Source: three-view drawing plus pictorial views. Frame: mm from the lowest corner of the part. A direction names the side the tool comes from. Coordinates: 2 decimals unless noted, no trailing zeros. Order: outer loops, then holes, each group sorted by start corner. A loop starts at its lowest first (then second) coordinate and runs counter-clockwise, first axis right, second up. Notation, with made-up numbers: (69, -27.75) -> (84, -27.75) arc R15 ccw to (84, -15.75) -> close; hole circle Ø11 at (3, 19). An arc over 180 degrees is marked (long way). Use one line per item in the form item = value. Start each with the question number.
1) Pin query (flat end, axial travel): pin 1 (4 mm diameter, centred on y = 4.5, z = 7, fed in from -X); pin 2 (6.5 mm diameter, centred on x = 9.5, y = 7, fed in from +Z); pin 3 (2 mm diameter, centred on x = 5.5, z = 3, fed in from +Y); pin 4 (5 mm diameter, centred on y = 12.5, z = 4, fed in from +X). Return the tip coordinate at first contact, or that it passes through.
2) Ray query, line 1 along Y through (x, z) = (8, 9.5); line 2 along Z through (x, y) = (2, 12.25); line 3 along Z through (x, y) = (4.25, 7.25). Return the intervals inside material, ascending.
3) Access query for the marked faces 4 and 5. Directions: +Z, -Z, +X, -X, +Y, -Y. A direction counts if a zero-diameter tool reaches every point of the face in a straight line with its end or side. Return the directions, or none.
4) Section query C-C on z = 8. Output: boundary loops of the cut face in (x, y), then the cut area to 3 significant figures.
5) Draft query along X for the marked faces 1, 2 and 3. Return one class per face: pulls with the +X half, pulls with the -X half, needs draft (parallel to the pull), parting line crosses it, or undercut.
6) Section query D-D on z = 2.75. Output: boundary loops of the cut face in (x, y), then the cut area to 3 significant figures.
7) Section query A-A on y = 8. Output: boundary loops of the cut face in (x, z), then the cut area to 3 significant figures.
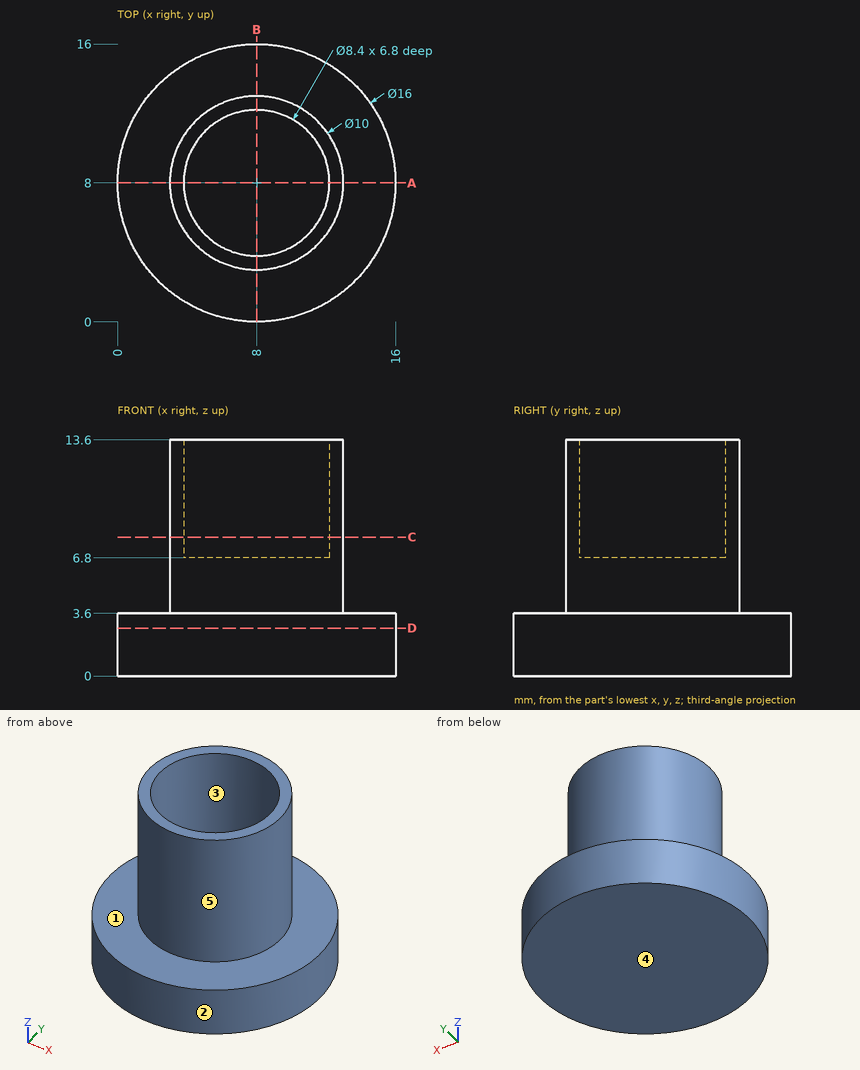
Answers below:
q1.pin_1 = 3.23
q1.pin_2 = 13.6
q1.pin_3 = 15.86
q1.pin_4 = 15.74
q2.line_1 = 3 to 3.8, 12.2 to 13
q2.line_2 = 0 to 3.6
q2.line_3 = 0 to 6.8
q3.face_4 = -Z, +X, -X, +Y, -Y
q3.face_5 = +Z
q4.outline = circle Ø10 at (8, 8); hole circle Ø8.4 at (8, 8)
q4.area = 23.1 mm^2
q5.face_1 = needs draft
q5.face_2 = parting line crosses it
q5.face_3 = undercut
q6.outline = circle Ø16 at (8, 8)
q6.area = 201 mm^2
q7.outline = (0, 0) -> (16, 0) -> (16, 3.6) -> (13, 3.6) -> (13, 13.6) -> (12.2, 13.6) -> (12.2, 6.8) -> (3.8, 6.8) -> (3.8, 13.6) -> (3, 13.6) -> (3, 3.6) -> (0, 3.6) -> close
q7.area = 100 mm^2
